Check sheet for the drawn part. Datum: minimum x, y, z corner. Units: mm. Coordinates: 2 decimals unless noted, no trailing zeros.
Q1. Depth check by flat-ended pin: P1, Ø4.5, axis at x = 5.55, z = 31.5, coming from the +Y side; P2, Ø7.5, axis at x = 37, z = 31, coming from the +Y side; P3, Ø5, axis at x = 13, y = 3, coming from the -Z side. Enter the tip coordinate at first touch or a pass-through.
Q2. Thickness scan on line 1 (Y direction, x = 23.5, z = 40); line 2 (X direction, y = 1, z = 24.5); line 3 (X direction, y = 3.75, z = 26) (1 decimal). Record the ranges inside material, lowest first.
Q3. Cross-section at A-A, the plane x = 22. Count the separate pieces of the cut face and the enclosed holes in it, and give its area (3 significant figures).
Q4. Draft check along Z on the marked faces 1, 2, 3 and 4. Enter one of: pulls with the +Z half, pulls with the -Z half, needs draft (parallel to the pull), parting line crosses it, or undercut.
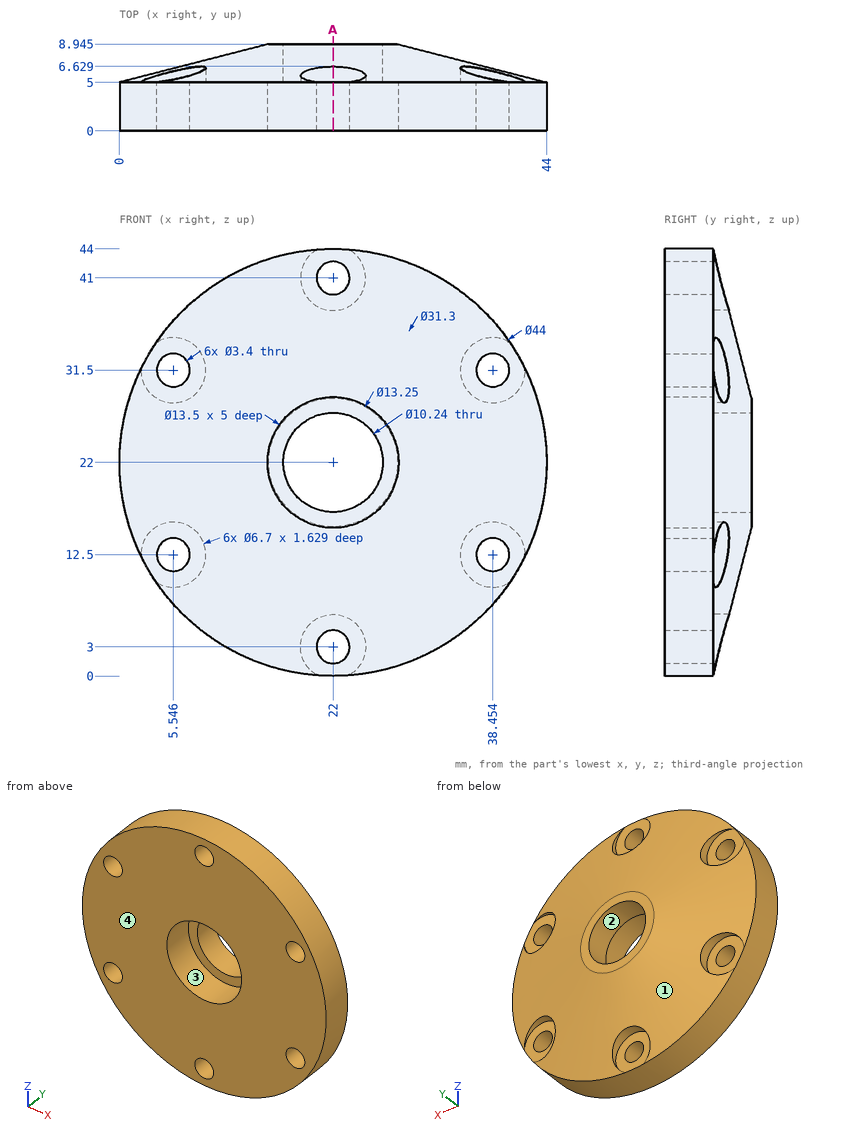
Check values:
1. P1: stops at y = 5
1. P2: stops at y = 7.12
1. P3: stops at z = 0.98
2. line 1: y = 0 to 5
2. line 2: x = 0.14 to 15.73, 28.27 to 43.86
2. line 3: x = 0.4 to 16.6, 27.4 to 43.6
3. separate pieces: 4
3. enclosed holes: 0
3. area: 181 mm2
4. face 1: parting line crosses it
4. face 2: undercut
4. face 3: undercut
4. face 4: needs draft
